The model under review builds one solid part; all positions refer to its coordinate system, in mm. A direction names the side the tool comes from. Give positions to 0.01 mm unless a question says otherwise; leave off trailing zeros. Order: outer loops, then holes, each group sorted by start corner. A loop starts at its lowest first (then second) coordinate and runs counter-clockwise, first axis right, second up. Notation, with made-up numbers: (-30.75, 71.25) - (11.25, 71.25) arc R29 cw to (11.25, 97.25) - close; hole circle Ø2 at (-12, 52). An arc over 180 degrees is marked (long way). Write item = value, one per line. Start each with the question number.
1. Wall thickness on probe 1 along Y at (x, z) = (-67.5, -21.5); probe 2 along Y at (x, z) = (-66.5, -35); probe 3 along X at (y, z) = (74, -32.5): over which ranges is each line inside the solid? List them lowest first.
2. For P1, Ø6, axis at y = 39.5, z = -16, coming from the -X side; P2, Ø12, axis at y = 121.5, z = -15.5, coming from the -X side; P3, Ø2, axis at x = -88, y = 91.5, coming from the -Z side; P4, Ø10, axis at x = -89, z = -5, coming from the -Y side, all flat-tipped, find the tip position at first contact; note any pin that passes through.
3. We need section A-A, the plane y = 112.5. Give the boundary of the cut face in (x, z), and give its area (3 significant figures).
4. We need section B-B, the plane y = 69.5. Give the boundary of the cut face in (x, z), and give its area (3 significant figures).
5. Machinability: for faces 1 (the flat face through (-73, 0, -16)), 2 (the cylindrical face through (-76.215, 147.185, -15.412)), 3 (the cylindrical face through (-93.1, 74.78, -5.09)), which of the approach directions +Z, -Z, +X, -X, +Y, -Y give a long, thin tool a straight path to every point of the face, cutting with its end or side? Answer none if there is none.
from build123d import *

# Parameters (mm, degrees)
SKETCH1_R           = 19
BOSS_EXTRUDE1_DEPTH = 57
SKETCH2_R           = 23.5
BOSS_EXTRUDE2_DEPTH = 34
SKETCH3_R           = 27.5
SKETCH4_R           = 23.5
SKETCH5_R           = 4
BOSS_EXTRUDE3_DEPTH = 45
FILLET1_R           = 2


with BuildPart() as part:
    # Sketch1 → Boss-Extrude1 (new body)
    with BuildSketch(Plane(origin=(0, 0, 0), x_dir=(1, 0, 0), z_dir=(0, 1, 0))):
        with Locations(Location((-72.248941829, 15.932254861, 0), (0, 0, 90))):
            Circle(SKETCH1_R)
    extrude(amount=BOSS_EXTRUDE1_DEPTH)

    # Sketch2 → Boss-Extrude2 (add)
    with BuildSketch(Plane(origin=(0, 57, 0), x_dir=(1, 0, 0), z_dir=(0, 1, 0))):
        with Locations(Location((-72.248941829, 15.932254861, 0), (0, 0, 270))):
            Circle(SKETCH2_R)
    extrude(amount=BOSS_EXTRUDE2_DEPTH)

    # Sketch3 → Loft1 section 0
    with BuildSketch(Plane(origin=(0, 91, 0), x_dir=(1, 0, 0), z_dir=(0, 1, 0))):
        with Locations((-72.248941829, 15.932254861)):
            Circle(SKETCH3_R)
    # Sketch4 → Loft1 section 1
    with BuildSketch(Plane(origin=(0, 125, 0), x_dir=(1, 0, 0), z_dir=(0, 1, 0))):
        with Locations((-72.248941829, 15.932254861)):
            Circle(SKETCH4_R)
    loft()

    # Sketch5 → Boss-Extrude3 (add)
    with BuildSketch(Plane(origin=(0, 125, 0), x_dir=(1, 0, 0), z_dir=(0, 1, 0))):
        with Locations(Location((-72.248941829, 15.932254861, 0), (0, 0, 90))):
            Circle(SKETCH5_R)
    extrude(amount=BOSS_EXTRUDE3_DEPTH)

    # Fillet1
    fillet1_edges = [part.edges().sort_by_distance(p)[0] for p in [
        (-95.748941829, 125, -15.932254861),
        (-99.748941829, 91, -15.932254861),
        (-72.248941829, 57, -39.432254861),
    ]]
    fillet(fillet1_edges, radius=FILLET1_R)


solid = part.part
Model answer:
q1.probe_1 = 0 to 125
q1.probe_2 = 57 to 125
q1.probe_3 = -88.92 to -55.58
q2.P1 = -91.25
q2.P2 = -96.87
q2.P3 = -38.46
q2.P4 = 0
q3.outline = circle Ø49.94 at (-72.25, -15.93)
q3.area = 1,960 mm2
q4.outline = circle Ø47 at (-72.25, -15.93)
q4.area = 1,730 mm2
q5.face_1 = +Z, -Z, +X, -X, -Y
q5.face_2 = +Y
q5.face_3 = -Y
